from build123d import *

# Parameters (mm, degrees)
SKETCH1_R           = 1.5
BOSS_EXTRUDE1_DEPTH = 70
SKETCH2_W           = 4
SKETCH2_H           = 1.5
BOSS_EXTRUDE2_DEPTH = 5
SKETCH3_R           = 1
CUT_EXTRUDE1_DEPTH  = 3.25


with BuildPart() as part:
    # Sketch1 → Boss-Extrude1 (new body)
    with BuildSketch(Plane(origin=(0, 0, 0), x_dir=(1, 0, 0), z_dir=(0, 1, 0))):
        Circle(SKETCH1_R)
    extrude(amount=BOSS_EXTRUDE1_DEPTH)

    # Sketch2 → Boss-Extrude2 (add)
    with BuildSketch(Plane(origin=(0, 70, 0), x_dir=(1, 0, 0), z_dir=(0, 1, 0))):
        Rectangle(SKETCH2_W, SKETCH2_H)
    extrude(amount=BOSS_EXTRUDE2_DEPTH)

    # Sketch3 → Cut-Extrude1 (cut, through all)
    with BuildSketch(Plane(origin=(0, 0, -0.75), x_dir=(-1, 0, 0), z_dir=(0, 0, -1))):
        with Locations((0, 73)):
            Circle(SKETCH3_R)
    extrude(amount=-CUT_EXTRUDE1_DEPTH, mode=Mode.SUBTRACT)


solid = part.part
Check sheet for the modelled part. Datum: model origin and axes. Units: mm. A direction names the side the tool comes from. Round coordinates to 2 decimals unless told otherwise and drop trailing zeros. Order: outer loops, then holes, each group sorted by start corner. A loop starts at its lowest first (then second) coordinate and runs counter-clockwise, first axis right, second up. Notation, with made-up numbers: M 5,-38 L 13,-38 A20 ccw 13,-10 Z; hole C 50.25,-29 d6. An arc over 180 degrees is marked long. One line per item, written item: value. Start each with the question number.
1. Scan lines: line 1 along Y through (x, z) = (0, 0.4); line 2 along X through (y, z) = (73, 0); line 3 along X through (y, z) = (23, 0.15). Record each from-to range of solid material in increasing order.
2. Section check D-D on y = 44. Enter the section's corners in (x, z).
3. Section check A-A on x = 0. Enter the section's corners in (y, z).
4. Gauge pin test, flat ends, axial feed: P1, Ø1, axis at y = 44, z = 1, coming from the +X side; P2, Ø1.2, axis at x = -0.5, y = 73, coming from the +Z side; P3, Ø2, axis at x = 0, y = 72.5, coming from the -Z side. Record the tip position at first contact, or that the pin passes through.
5. Release check for a two-part mould opening along X. For faces 4 (the flat face through (2, 72, 0)), 5 (the cylindrical face through (0, 72, 0)), 6 (the cylindrical face through (-1.5, 34.51, -0.07)) record: released by +X, released by -X, zero draft, split by the parting line, or undercut.
6. Section check B-B on z = 0. Enter the section's corners in (x, y), and give its area (3 significant figures).
7. Section check C-C on y = 73. Enter the section's corners in (x, z), and give its area (3 significant figures).
8. Access from +Z, -Z, +X, -X, +Y, -Y to the whole of each face (thin tool, end or side, straight path). Record for faces 1 (the flat face through (-0.5, 71.9, 0.75)), 2 (the flat face through (-2, 72, 0)), 3 (the flat face through (-0.5, 71.9, -0.75)).
Results found:
1. line 1: 0 to 72, 74 to 75
1. line 2: -2 to -1, 1 to 2
1. line 3: -1.49 to 1.49
2. outline: C 0,0 d3
3. outline: M 0,-1.5 L 70,-1.5 L 70,-0.75 L 72,-0.75 L 72,0.75 L 70,0.75 L 70,1.5 L 0,1.5 Z; M 74,-0.75 L 75,-0.75 L 75,0.75 L 74,0.75 Z
4. P1: x = 1.41
4. P2: z = 0.75
4. P3: z = -0.75
5. face 4: released by +X
5. face 5: undercut
5. face 6: split by the parting line
6. outline: M -2,70 L -1.5,70 L -1.5,0 L 1.5,0 L 1.5,70 L 2,70 L 2,75 L -2,75 Z; hole C 0,73 d2
6. area: 227 mm^2
7. outline: M -2,-0.75 L -1,-0.75 L -1,0.75 L -2,0.75 Z; M 1,-0.75 L 2,-0.75 L 2,0.75 L 1,0.75 Z
7. area: 3.00 mm^2
8. face 1: +Z, +X, -X, +Y
8. face 2: +Z, -Z, -X, +Y, -Y
8. face 3: -Z, +X, -X, +Y
